CAD build for the part. Positions are in the model's coordinates, mm. A direction names the side the tool comes from. Coordinates: 2 decimals unless noted, no trailing zeros. Loops run counter-clockwise (first coordinate to the right, second up) from the corner with the lowest first, then second, coordinate; pieces in that order, holes last. Notation, with made-up numbers: (-9, 26) - (44, 26) arc R9 cw to (44, 37) - close; hole circle Ø7 at (15.25, -0.75). An arc over 180 degrees is marked (long way). Put each result on its own line as item: value.
```python
from build123d import *

# Parameters (mm, degrees)
AUFSATZ_LINEAR_AUSTRAGEN1_DEPTH = 2
AUFSATZ_LINEAR_AUSTRAGEN5_DEPTH = 13
KREISMUSTER3_COUNT              = 3
KREISMUSTER3_ANGLE              = 120


with BuildPart() as part:
    # Skizze1 → Aufsatz-Linear austragen1 (new body)
    with BuildSketch(Plane.XY):
        with BuildLine():
            Line((29.011851027, 10.25), (28.145825623, 10.75))
            Line((28.145825623, 10.75), (25.547749412, 12.25))
            Line((25.547749412, 12.25), (21.217622393, 14.75))
            Line((21.217622393, 14.75), (18.619546181, 16.25))
            Line((18.619546181, 16.25), (17.753520778, 16.75))
            Line((17.753520778, 16.75), (16.454482672, 14.5))
            ThreePointArc((16.454482672, 14.5), (15.588457268, 14), (14.722431864, 14.5))
            Line((14.722431864, 14.5), (13.423393759, 16.75))
            Line((13.423393759, 16.75), (12.557368355, 16.25))
            Line((12.557368355, 16.25), (9.959292144, 14.75))
            Line((9.959292144, 14.75), (5.629165125, 12.25))
            Line((5.629165125, 12.25), (3.031088913, 10.75))
            Line((3.031088913, 10.75), (2.165063509, 10.25))
            Line((2.165063509, 10.25), (3.464101615, 8))
            ThreePointArc((3.464101615, 8), (3.464101615, 7), (2.598076211, 6.5))
            Line((2.598076211, 6.5), (0, 6.5))
            Line((0, 6.5), (0, 5.5))
            Line((0, 5.5), (0, 2.5))
            Line((0, 2.5), (0, -2.5))
            Line((0, -2.5), (0, -5.5))
            Line((0, -5.5), (0, -6.5))
            Line((0, -6.5), (4.330127019, -6.5))
            Line((4.330127019, -6.5), (6.92820323, -5))
            Line((6.92820323, -5), (24.248711306, 5))
            Line((24.248711306, 5), (26.846787517, 6.5))
            Line((26.846787517, 6.5), (29.011851027, 10.25))
        make_face()
    extrude(amount=AUFSATZ_LINEAR_AUSTRAGEN1_DEPTH)

    # Skizze6 → Aufsatz-Linear austragen5 (add)
    with BuildSketch(Plane.XZ.offset(6.5)):
        with BuildLine():
            Line((-48.004683363, 13), (-48.338732237, 11.105224302))
            ThreePointArc((-48.338732237, 11.105224302), (-24.026875813, 6.172842822), (0, 0))
            Line((0, 0), (0, 2))
            ThreePointArc((0, 2), (-23.862752465, 8.109176013), (-48.004683363, 13))
        make_face()
    aufsatz_linear_austragen5 = extrude(amount=-AUFSATZ_LINEAR_AUSTRAGEN5_DEPTH)

    # Kreismuster3: Aufsatz-Linear austragen5 ×3 about axis
    kreismuster3_axis = Axis((15.588457268, 0, 0), (0, 0, -1))
    for i in range(1, KREISMUSTER3_COUNT):
        add(aufsatz_linear_austragen5.rotate(kreismuster3_axis, i * KREISMUSTER3_ANGLE / (KREISMUSTER3_COUNT - 1)))


solid = part.part
```
Q1. Slice it at B-B, the plane y = 3. Give the cut face in (x, z), then the cut area to 3 significant figures.
Determined:
outline: (-48.34, 11.11) arc R483.51 cw to (0, 0) - (20.78, 0) - (20.78, 2) - (0, 2) arc R485.43 ccw to (-48, 13) - close
area: 137 mm2
Q2. Slice it at A-A, the plane z = 9.25. Give the cut face in (x, y), then the cut area to 3 significant figures.
Determined:
outline: (-38.42, -6.5) - (-28.97, -6.5) - (-28.97, 6.5) - (-38.42, 6.5) - close; (-17.05, 43.52) - (-12.32, 35.34) - (-1.06, 41.84) - (-5.79, 50.02) - close; (32.24, 41.84) - (43.5, 35.34) - (48.22, 43.52) - (36.96, 50.02) - close
area: 369 mm2
Q3. Mould opens along X. For faces 1 (the cylindrical face through (35.067, 33.92, 8.032)), 2 (the flat face through (-23, 6.5, 7)), 3 (the cylindrical face through (35.49, 34.65, 6.25)) say: +X half, -X half, draft (parallel to the pull), parting line (faces both ways), or undercut.
Determined:
face 1: undercut
face 2: draft
face 3: +X half
Q4. Wall check: L1, parallel to Y at x = -19, z = 5.25; L2, parallel to Y at x = -21, z = 12.25; L3, parallel to Z at x = -5, y = 23. Give the ranges that are in metal, low to high. Write a range as from..to.
Determined:
L1: -6.5..6.5
L2: 50.37..52.46
L3: 3.91..5.9
Q5. Pin check, flat tip, straight feed: pin 1 Ø4 at (x, z) = (-8, 10.5) entering from +Y. Stop position of the tip, or through.
Determined:
pin 1: y = 57.27
Q6. Tool access for faces 4 (the cylindrical face through (-4.048, 33.829, 8.032)), 5 (the flat face through (11, 5, 0)): list every direction of +Z, -Z, +X, -X, +Y, -Y with a clear straight run to the whole face (end or side of a thin tool).
Determined:
face 4: +Z, -Y
face 5: -Z, +X, -X, +Y, -Y
